```python
from build123d import *

# Parameters (mm, degrees)
SKETCH2_W           = 100
SKETCH2_H           = 80
BOSS_EXTRUDE1_DEPTH = 3
SKETCH3_W           = 3
SKETCH3_H           = 80
BOSS_EXTRUDE2_DEPTH = 100
SKETCH8_R           = 2
CUT_EXTRUDE3_DEPTH  = 61
SKETCH6_R           = 13
CUT_EXTRUDE4_DEPTH  = 10
SKETCH9_W           = 3
SKETCH9_H           = 80
CUT_EXTRUDE5_DEPTH  = 15


with BuildPart() as part:
    # Sketch2 → Boss-Extrude1 (new body)
    with BuildSketch(Plane(origin=(0, 0, 0), x_dir=(1, 0, 0), z_dir=(0, 1, 0))):
        Rectangle(SKETCH2_W, SKETCH2_H)
    extrude(amount=BOSS_EXTRUDE1_DEPTH)

    # Sketch3 → Boss-Extrude2 (add)
    with BuildSketch(Plane.XZ):
        with Locations((-48.5, 0)):
            Rectangle(SKETCH3_W, SKETCH3_H)
    extrude(amount=BOSS_EXTRUDE2_DEPTH)

    # Sketch8 → Cut-Extrude3 (cut)
    with BuildSketch(Plane(origin=(0, 3, 0), x_dir=(1, 0, 0), z_dir=(0, 1, 0))):
        with Locations((-30, 20)):
            Circle(SKETCH8_R)
        with Locations((-30, -20)):
            Circle(SKETCH8_R)
    extrude(amount=-CUT_EXTRUDE3_DEPTH, mode=Mode.SUBTRACT)

    # Sketch6 → Cut-Extrude4 (cut)
    with BuildSketch(Plane.ZY.offset(50)):
        with Locations((0, -51.5)):
            Circle(SKETCH6_R)
    extrude(amount=-CUT_EXTRUDE4_DEPTH, mode=Mode.SUBTRACT)

    # Sketch9 → Cut-Extrude5 (cut)
    with BuildSketch(Plane.XZ.offset(100)):
        with Locations((-48.5, 0)):
            Rectangle(SKETCH9_W, SKETCH9_H)
    extrude(amount=-CUT_EXTRUDE5_DEPTH, mode=Mode.SUBTRACT)


solid = part.part
```
Source: CAD feature listing. Evaluate the final solid. Frame: model axes, mm. A direction names the side the tool comes from. Coordinates: 2 decimals unless noted, no trailing zeros. Loops run counter-clockwise (first coordinate to the right, second up) from the corner with the lowest first, then second, coordinate; pieces in that order, holes last. Notation, with made-up numbers: M 4,72.5 L 15,72.5 A32 ccw 15,102.5 Z; hole C -24.75,42.25 d9. An arc over 180 degrees is marked long. Put each result on its own line as item: value. Start each with the question number.
1) Pull-direction query (Z, two-part tool) for faces 1 (the face through (-48.52, -38.61, -1.69)), 2 (the face through (1, 0, -1)), 3 (the face through (-22, 2, 40)), 4 (the face through (-22, 2, -40)); classes: pulls with the +Z half, pulls with the -Z half, needs draft (parallel to the pull), parting line crosses it, or undercut.
2) Ray query, L1, parallel to Z at x = -30, y = 2; L2, parallel to Y at x = -49, z = 0; L3, parallel to X at y = 1.7, z = 20. Return the intervals inside material, ascending. Write a range as from..to.
3) Cut plane C-C on x = -30. Return the cut outline in (y, z), then the cut area to 3 significant figures.
4) Reachability of faces 5 (the face through (-47, -32, -1)), 6 (the face through (-28.092, 1.521, -20.601)) from +Z, -Z, +X, -X, +Y, -Y: full face, straight path, thin tool, end or side. Return the list, or none.
5) Cut plane A-A on z = 0. Return the cut outline in (x, y), then the cut area to 3 significant figures.
6) Cut plane D-D on z = 20. Return the cut outline in (x, y).
7) Cut plane B-B on y = -51.5. Return the cut outline in (x, z), then the cut area to 3 significant figures.
8) Contact query for flat-ended pins moving along their axis: pin 1 Ø6 at (y, z) = (-67, 0.5) entering from +X; pin 2 Ø6.5 at (x, z) = (-30, -20) entering from -Y; pin 3 Ø23.5 at (y, z) = (-51.5, 0) entering from -X. Output: stop coordinate, or through.
The answers:
1. face 1: undercut
1. face 2: needs draft
1. face 3: pulls with the +Z half
1. face 4: pulls with the -Z half
2. L1: z = -40..-22, -18..18, 22..40
2. L2: y = -85..-64.5, -38.5..3
2. L3: x = -50..-32, -28..50
3. outline: M 0,-40 L 3,-40 L 3,-22 L 0,-22 Z; M 0,-18 L 3,-18 L 3,18 L 0,18 Z; M 0,22 L 3,22 L 3,40 L 0,40 Z
3. area: 216 mm²
4. face 5: +Z, -Z, +X, -Y
4. face 6: +Y, -Y
5. outline: M -50,-85 L -47,-85 L -47,-64.5 L -50,-64.5 Z; M -50,-38.5 L -47,-38.5 L -47,0 L 50,0 L 50,3 L -50,3 Z
5. area: 477 mm²
6. outline: M -50,-85 L -47,-85 L -47,0 L -32,0 L -32,3 L -50,3 Z; M -28,0 L 50,0 L 50,3 L -28,3 Z
7. outline: M -50,-40 L -47,-40 L -47,-13 L -50,-13 Z; M -50,13 L -47,13 L -47,40 L -50,40 Z
7. area: 162 mm²
8. pin 1: stops at x = -47
8. pin 2: stops at y = 0
8. pin 3: passes through
